Could you check a few things on this model? Use its own coordinates, in mm. A direction names the side the tool comes from. Coordinates: 2 decimals unless noted, no trailing zeros. Loops run counter-clockwise (first coordinate to the right, second up) from the corner with the lowest first, then second, coordinate; pieces in that order, holes last. Notation, with made-up numbers: (13.5, 2) - (22.5, 2) arc R20 cw to (22.5, 33) - close; hole circle Ø5 at (18.5, 87). An arc over 180 degrees is marked (long way). Use CSV: the item, a comma, the result in double quotes.
Autodesk Fusion 360 part; units mm, degrees
sketch "Sketch1" plane through (0, 0, 0) normal (0, 0, 1) x (1, 0, 0)
  line L0 (30, -30) -> (-30, -30)
  line L1 (-30, -30) -> (-30, 30)
  line L2 (-30, 30) -> (30, 30)
  line L3 (30, 30) -> (30, -30)
  line L4 (30, -30) -> (-30, 30) construction
  line L5 (-30, -30) -> (30, 30) construction
  dimension "d1" = 60
  dimension "d2" = 60
extrude "Extrude1" add sketch "Sketch1" along normal blind 6.35
sketch "Sketch2" plane through (0, 0, 6.35) normal (0, 0, 1) x (1, 0, 0)
  line L0 (30, 30) -> (-30, 30)
  line L1 (-30, 30) -> (-30, -30)
  line L2 (-30, -30) -> (30, -30)
  line L3 (30, -30) -> (30, 30)
  line L4 (20.5, -20.5) -> (-20.5, -20.5)
  line L5 (-20.5, -20.5) -> (-20.5, 20.5)
  line L6 (-20.5, 20.5) -> (20.5, 20.5)
  line L7 (20.5, 20.5) -> (20.5, -20.5)
  line L8 (20.5, -20.5) -> (-20.5, 20.5) construction
  line L9 (-20.5, -20.5) -> (20.5, 20.5) construction
  circle A0 centre (-20.5, 20.5) radius 3.575
  circle A1 centre (20.5, 20.5) radius 3.575
  circle A2 centre (20.5, -20.5) radius 2.5
  circle A3 centre (-20.5, -20.5) radius 2.5
  dimension "d5" = 41
  dimension "d6" = 41
  dimension "d7" = 7.15
  dimension "d8" = 7.15
  dimension "d9" = 5
  dimension "d10" = 5
extrude "Extrude2" cut sketch "Sketch2" against normal through all contours L4 L5 A3 | L4 L5 A3 | L4 L7 A2 | L4 L7 A2 | L5 L6 A0 | L5 L6 A0 | L6 L7 A1 | L6 L7 A1
sketch "Sketch3" plane through (0, 0, 6.35) normal (0, 0, 1) x (1, 0, 0)
  circle A0 centre (-20.5, -20.5) radius 2.5
  circle A1 centre (-20.5, 20.5) radius 3.575
  circle A2 centre (20.5, -20.5) radius 2.5
  circle A3 centre (20.5, 20.5) radius 3.575
  line L0 (30, 30) -> (-30, 30)
  line L1 (-30, 30) -> (-30, -30)
  line L2 (-30, -30) -> (30, -30)
  line L3 (30, -30) -> (30, 30)
  circle A4 centre (-20.5, -20.5) radius 5.05
  circle A5 centre (20.5, -20.5) radius 5.05
  circle A6 centre (20.5, 20.5) radius 5.05
  circle A7 centre (-20.5, 20.5) radius 5.05
  dimension "d12" = 10.1
  dimension "d13" = 10.1
  dimension "d14" = 10.1
  dimension "d15" = 10.1
extrude "Extrude3" cut sketch "Sketch3" against normal blind 2 contours A4 | A5 | A6 | A7
fillet "Fillet1" radius 5 2 edges at (30, -30, 3.175) (30, 30, 3.175)
fillet "Fillet2" radius 5 2 edges at (-30, 30, 3.175) (-30, -30, 3.175)
sketch "Sketch4" plane through (0, 0, 6.35) normal (0, 0, 1) x (1, 0, 0)
  arc A0 (-30, -25) -> (-25, -30) centre (-25, -25) ccw
  line L0 (-25, -30) -> (25, -30)
  arc A1 (25, -30) -> (30, -25) centre (25, -25) ccw
  line L1 (30, -25) -> (30, 25)
  arc A2 (30, 25) -> (25, 30) centre (25, 25) ccw
  line L2 (25, 30) -> (-25, 30)
  arc A3 (-25, 30) -> (-30, 25) centre (-25, 25) ccw
  line L3 (-30, 25) -> (-30, -25)
  circle A4 centre (20.5, 20.5) radius 5.05
  circle A5 centre (20.5, -20.5) radius 5.05
  circle A6 centre (-20.5, 20.5) radius 5.05
  circle A7 centre (-20.5, -20.5) radius 5.05
  circle A8 centre (0, 0) radius 2.5
  circle A9 centre (10, 0) radius 2.5
  circle A10 centre (-10, 0) radius 2.5
  line L4 (-25.75, -3.375) -> (-28.25, -3.375)
  line L5 (-28.25, -3.375) -> (-28.25, 3.375)
  line L6 (-28.25, 3.375) -> (-25.75, 3.375)
  line L7 (-25.75, 3.375) -> (-25.75, -3.375)
  line L8 (-25.75, -3.375) -> (-28.25, 3.375) construction
  line L9 (-28.25, -3.375) -> (-25.75, 3.375) construction
  line L10 (28.25, -3.375) -> (25.75, -3.375)
  line L11 (25.75, -3.375) -> (25.75, 3.375)
  line L12 (25.75, 3.375) -> (28.25, 3.375)
  line L13 (28.25, 3.375) -> (28.25, -3.375)
  line L14 (28.25, -3.375) -> (25.75, 3.375) construction
  line L15 (25.75, -3.375) -> (28.25, 3.375) construction
  point P0 (-27, 0)
  point P1 (27, 0)
  dimension "d20" = 5
  dimension "d21" = 5
  dimension "d22" = 5
  dimension "d23" = 6.75
  dimension "d24" = 2.5
  dimension "d25" = 6.75
  dimension "d26" = 2.5
extrude "Extrude4" cut sketch "Sketch4" against normal through all contours A8 | A9 | A10 | L4 L5 L6 L7 | L10 L11 L12 L13
sketch "Sketch5" plane through (0, 0, 6.35) normal (0, 0, 1) x (1, 0, 0)
  circle A0 centre (0, 0) radius 2.5
  circle A1 centre (-10, 0) radius 2.5
  circle A2 centre (10, 0) radius 2.5
  line L0 (-25.75, 3.375) -> (-25.75, -3.375)
  line L1 (-25.75, -3.375) -> (-28.25, -3.375)
  line L2 (-28.25, -3.375) -> (-28.25, 3.375)
  line L3 (-28.25, 3.375) -> (-25.75, 3.375)
  line L4 (28.25, 3.375) -> (28.25, -3.375)
  line L5 (28.25, -3.375) -> (25.75, -3.375)
  line L6 (25.75, -3.375) -> (25.75, 3.375)
  line L7 (25.75, 3.375) -> (28.25, 3.375)
  arc A3 (-30, -25) -> (-25, -30) centre (-25, -25) ccw
  line L8 (-25, -30) -> (25, -30)
  arc A4 (25, -30) -> (30, -25) centre (25, -25) ccw
  line L9 (30, -25) -> (30, 25)
  arc A5 (30, 25) -> (25, 30) centre (25, 25) ccw
  line L10 (25, 30) -> (-25, 30)
  arc A6 (-25, 30) -> (-30, 25) centre (-25, 25) ccw
  line L11 (-30, 25) -> (-30, -25)
  circle A7 centre (20.5, 20.5) radius 5.05
  circle A8 centre (20.5, -20.5) radius 5.05
  circle A9 centre (-20.5, 20.5) radius 5.05
  circle A10 centre (-20.5, -20.5) radius 5.05
  circle A11 centre (-20.5, 20.5) radius 6
  circle A12 centre (20.5, 20.5) radius 6
  dimension "d28" = 12
  dimension "d29" = 12
extrude "Extrude5" cut sketch "Sketch5" against normal blind 2 contours A11 | A12
sketch "Sketch6" plane through (0, 0, 6.35) normal (0, 0, 1) x (1, 0, 0)
  circle A0 centre (-20.5, 20.5) radius 6
  circle A1 centre (20.5, 20.5) radius 6
  circle A2 centre (0, 0) radius 2.5
  circle A3 centre (-10, 0) radius 2.5
  circle A4 centre (10, 0) radius 2.5
  line L0 (-25.75, 3.375) -> (-25.75, -3.375)
  line L1 (-25.75, -3.375) -> (-28.25, -3.375)
  line L2 (-28.25, -3.375) -> (-28.25, 3.375)
  line L3 (-28.25, 3.375) -> (-25.75, 3.375)
  line L4 (28.25, 3.375) -> (28.25, -3.375)
  line L5 (28.25, -3.375) -> (25.75, -3.375)
  line L6 (25.75, -3.375) -> (25.75, 3.375)
  line L7 (25.75, 3.375) -> (28.25, 3.375)
  arc A5 (-30, -25) -> (-25, -30) centre (-25, -25) ccw
  line L8 (-25, -30) -> (25, -30)
  arc A6 (25, -30) -> (30, -25) centre (25, -25) ccw
  line L9 (30, -25) -> (30, 25)
  arc A7 (30, 25) -> (25, 30) centre (25, 25) ccw
  line L10 (25, 30) -> (-25, 30)
  arc A8 (-25, 30) -> (-30, 25) centre (-25, 25) ccw
  line L11 (-30, 25) -> (-30, -25)
  circle A9 centre (20.5, -20.5) radius 5.05
  circle A10 centre (-20.5, -20.5) radius 5.05
  circle A11 centre (-20.5, 20.5) radius 3.65
  circle A12 centre (20.5, 20.5) radius 3.65
  dimension "d32" = 7.3
  dimension "d33" = 7.3
extrude "Extrude6" cut sketch "Sketch6" against normal through all contours A11
sketch "Sketch7" plane through (0, 0, 4.35) normal (0, 0, 1) x (1, 0, 0)
  circle A0 centre (20.5, 20.5) radius 6
  circle A1 centre (20.5, 20.5) radius 3.575
  circle A2 centre (20.5, 20.5) radius 3.65
  dimension "d35" = 7.3
extrude "Extrude7" cut sketch "Sketch7" against normal through all contours A2
move_face "OffsetFaces1" offset -1 1 faces at (-25.75, 1.125, 4.2333)
move_face "OffsetFaces2" offset 1 1 faces at (28.25, -1.125, 2.1167)
move_face "OffsetFaces3" offset 1 1 faces at (-28.25, 1.125, 2.1167)
move_face "OffsetFaces4" offset -1 1 faces at (25.75, 1.125, 2.1167)
sketch "Sketch9" plane through (0, 0, 6.35) normal (0, 0, 1) x (1, 0, 0)
  circle A0 centre (-20.5, 20.5) radius 6
  circle A1 centre (20.5, 20.5) radius 6
  circle A2 centre (0, 0) radius 2.5
  circle A3 centre (-10, 0) radius 2.5
  circle A4 centre (10, 0) radius 2.5
  line L0 (-24.75, 3.375) -> (-24.75, -3.375)
  line L1 (-24.75, -3.375) -> (-27.25, -3.375)
  line L2 (-27.25, -3.375) -> (-27.25, 3.375)
  line L3 (-27.25, 3.375) -> (-24.75, 3.375)
  line L4 (27.25, 3.375) -> (27.25, -3.375)
  line L5 (27.25, -3.375) -> (24.75, -3.375)
  line L6 (24.75, -3.375) -> (24.75, 3.375)
  line L7 (24.75, 3.375) -> (27.25, 3.375)
  arc A5 (-30, -25) -> (-25, -30) centre (-25, -25) ccw
  line L8 (-25, -30) -> (25, -30)
  arc A6 (25, -30) -> (30, -25) centre (25, -25) ccw
  line L9 (30, -25) -> (30, 25)
  arc A7 (30, 25) -> (25, 30) centre (25, 25) ccw
  line L10 (25, 30) -> (-25, 30)
  arc A8 (-25, 30) -> (-30, 25) centre (-25, 25) ccw
  line L11 (-30, 25) -> (-30, -25)
  circle A9 centre (20.5, -20.5) radius 5.05
  circle A10 centre (-20.5, -20.5) radius 5.05
  line L12 (-27.25, 3.375) -> (-30, 3.375)
  line L13 (-30, 3.375) -> (-30, -3.375)
  line L14 (-30, -3.375) -> (-27.25, -3.375)
  line L15 (-27.25, -3.375) -> (-27.25, 3.375)
  circle A11 centre (-0.0171, 20.5) radius 3.625
  dimension "d48" = 6.75
  dimension "d51" = 7.25
extrude "Extrude9" cut sketch "Sketch9" against normal blind 1.75 contours L2 L11 L12 L13 L14 L15
sketch "Sketch10" plane through (0, 0, 6.35) normal (0, 0, 1) x (1, 0, 0)
  line L0 (-30, -3.375) -> (-30, -25)
  arc A0 (-30, -25) -> (-25, -30) centre (-25, -25) ccw
  line L1 (-25, -30) -> (25, -30)
  arc A1 (25, -30) -> (30, -25) centre (25, -25) ccw
  line L2 (30, -25) -> (30, 25)
  arc A2 (30, 25) -> (25, 30) centre (25, 25) ccw
  line L3 (25, 30) -> (-25, 30)
  arc A3 (-25, 30) -> (-30, 25) centre (-25, 25) ccw
  line L4 (-30, 25) -> (-30, 3.375)
  line L5 (-30, 3.375) -> (-24.75, 3.375)
  line L6 (-24.75, 3.375) -> (-24.75, -3.375)
  line L7 (-24.75, -3.375) -> (-30, -3.375)
  circle A4 centre (-20.5, 20.5) radius 6
  circle A5 centre (20.5, 20.5) radius 6
  circle A6 centre (0, 0) radius 2.5
  circle A7 centre (-10, 0) radius 2.5
  circle A8 centre (10, 0) radius 2.5
  line L8 (27.25, 3.375) -> (27.25, -3.375)
  line L9 (27.25, -3.375) -> (24.75, -3.375)
  line L10 (24.75, -3.375) -> (24.75, 3.375)
  line L11 (24.75, 3.375) -> (27.25, 3.375)
  circle A9 centre (20.5, -20.5) radius 5.05
  circle A10 centre (-20.5, -20.5) radius 5.05
  line L12 (27.25, 3.375) -> (30, 3.375)
  line L13 (30, 3.375) -> (30, -3.375)
  line L14 (30, -3.375) -> (27.25, -3.375)
  line L15 (27.25, -3.375) -> (27.25, 3.375)
  dimension "d45" = 6.75
extrude "Extrude10" cut sketch "Sketch10" against normal blind 1.75 contours L2 L8 L12 L13 L14 L15
extrude "Extrude11" cut sketch "Sketch9" against normal blind 1.75 contours L2 L11 L12 L13 L14 L15
extrude "Extrude12" cut sketch "Sketch9" against normal through all contours A11
sketch "Sketch11" plane through (0, 0, 6.35) normal (0, 0, 1) x (1, 0, 0)
  circle A0 centre (-0.0171, 20.5) radius 3.625
  line L0 (30, -3.375) -> (24.75, -3.375)
  line L1 (24.75, -3.375) -> (24.75, 3.375)
  line L2 (24.75, 3.375) -> (30, 3.375)
  line L3 (30, 3.375) -> (30, 25)
  arc A1 (30, 25) -> (25, 30) centre (25, 25) ccw
  line L4 (25, 30) -> (-25, 30)
  arc A2 (-25, 30) -> (-30, 25) centre (-25, 25) ccw
  line L5 (-30, 25) -> (-30, 3.375)
  line L6 (-30, 3.375) -> (-24.75, 3.375)
  line L7 (-24.75, 3.375) -> (-24.75, -3.375)
  line L8 (-24.75, -3.375) -> (-30, -3.375)
  line L9 (-30, -3.375) -> (-30, -25)
  arc A3 (-30, -25) -> (-25, -30) centre (-25, -25) ccw
  line L10 (-25, -30) -> (25, -30)
  arc A4 (25, -30) -> (30, -25) centre (25, -25) ccw
  line L11 (30, -25) -> (30, -3.375)
  circle A5 centre (-20.5, -20.5) radius 5.05
  circle A6 centre (20.5, -20.5) radius 5.05
  circle A7 centre (10, 0) radius 2.5
  circle A8 centre (-10, 0) radius 2.5
  circle A9 centre (0, 0) radius 2.5
  circle A10 centre (20.5, 20.5) radius 6
  circle A11 centre (-20.5, 20.5) radius 6
  circle A12 centre (-0.0171, 20.5) radius 6
  dimension "d53" = 12
extrude "Extrude13" cut sketch "Sketch11" against normal blind 2 contours A12
sketch "Sketch12" plane through (0, 0, 6.35) normal (0, 0, 1) x (1, 0, 0)
  circle A0 centre (-0.0171, 20.5) radius 6
  line L0 (30, -3.375) -> (24.75, -3.375)
  line L1 (24.75, -3.375) -> (24.75, 3.375)
  line L2 (24.75, 3.375) -> (30, 3.375)
  line L3 (30, 3.375) -> (30, 25)
  arc A1 (30, 25) -> (25, 30) centre (25, 25) ccw
  line L4 (25, 30) -> (-25, 30)
  arc A2 (-25, 30) -> (-30, 25) centre (-25, 25) ccw
  line L5 (-30, 25) -> (-30, 3.375)
  line L6 (-30, 3.375) -> (-24.75, 3.375)
  line L7 (-24.75, 3.375) -> (-24.75, -3.375)
  line L8 (-24.75, -3.375) -> (-30, -3.375)
  line L9 (-30, -3.375) -> (-30, -25)
  arc A3 (-30, -25) -> (-25, -30) centre (-25, -25) ccw
  line L10 (-25, -30) -> (25, -30)
  arc A4 (25, -30) -> (30, -25) centre (25, -25) ccw
  line L11 (30, -25) -> (30, -3.375)
  circle A5 centre (-20.5, -20.5) radius 5.05
  circle A6 centre (20.5, -20.5) radius 5.05
  circle A7 centre (10, 0) radius 2.5
  circle A8 centre (-10, 0) radius 2.5
  circle A9 centre (0, 0) radius 2.5
  circle A10 centre (20.5, 20.5) radius 6
  circle A11 centre (-20.5, 20.5) radius 6
(1) Suppose I cut it at D-D (z = 3). State how many separate pieces and enclosed holes the cut face has, plus the area to 3 significant figures.
Computed:
separate pieces,"1"
enclosed holes,"10"
area,"3,320 mm²"
(2) Suppose I cut it at A-A (x = -20.5). Write out the boundary of the cut face in (y, z), plus the area to 3 significant figures.
Computed:
outline,"(-30, 0) - (-23, 0) - (-23, 4.35) - (-25.55, 4.35) - (-25.55, 6.35) - (-30, 6.35) - close; (-18, 0) - (16.85, 0) - (16.85, 4.35) - (14.5, 4.35) - (14.5, 6.35) - (-15.45, 6.35) - (-15.45, 4.35) - (-18, 4.35) - close; (24.15, 0) - (30, 0) - (30, 6.35) - (26.5, 6.35) - (26.5, 4.35) - (24.15, 4.35) - close"
area,"283 mm²"
(3) Which directions (+Z, -Z, +X, -X, +Y, -Y) give clear straight access to the entire face, cutting with the end or side of a thin tool? Please do faces 5 (the face through (0, -6, 6.35)), 6 (the face through (18, -22, 4.35)), 7 (the face through (-29, 0, 4.6)), 8 (the face through (27.25, 0, 2)), 9 (the face through (29, 0, 4.6)).
Computed:
face 5,"+Z, +X, -X, +Y, -Y"
face 6,"+Z"
face 7,"+Z, -X"
face 8,"+Z, -Z"
face 9,"+Z, +X"
(4) Suppose I cut it at B-B (x = -10). Write out the boundary of the cut face in (y, z).
Computed:
outline,"(-30, 0) - (-2.5, 0) - (-2.5, 6.35) - (-30, 6.35) - close; (2.5, 0) - (30, 0) - (30, 6.35) - (2.5, 6.35) - close"
(5) Thinking about a two-plate mould opening in Y: for faces 1 (the face through (0, 30, 3)), 2 (the face through (28, -29, 3)), 3 (the face through (1.656, 17.284, 2.205)), 4 (the face through (-30, 0, 3)), which applies, +Y half, -Y half, draft (parallel to the pull), parting line (faces both ways), or undercut?
Computed:
face 1,"+Y half"
face 2,"-Y half"
face 3,"undercut"
face 4,"draft"
(6) Suppose I cut it at C-C (y = 20.5). Write out the boundary of the cut face in (x, z), plus the area to 3 significant figures.
Computed:
outline,"(-30, 0) - (-24.15, 0) - (-24.15, 4.35) - (-26.5, 4.35) - (-26.5, 6.35) - (-30, 6.35) - close; (-16.85, 0) - (-3.64, 0) - (-3.64, 4.35) - (-6.02, 4.35) - (-6.02, 6.35) - (-14.5, 6.35) - (-14.5, 4.35) - (-16.85, 4.35) - close; (3.61, 0) - (16.85, 0) - (16.85, 4.35) - (14.5, 4.35) - (14.5, 6.35) - (5.98, 6.35) - (5.98, 4.35) - (3.61, 4.35) - close; (24.15, 0) - (30, 0) - (30, 6.35) - (26.5, 6.35) - (26.5, 4.35) - (24.15, 4.35) - close"
area,"214 mm²"
(7) Will these pins go through, and if not, where does the flat tip stop? pin 1 (14 mm diameter, centred on x = -0.02, y = 20.5, fed in from +Z); pin 2 (1.6 mm diameter, centred on x = 26, z = 3.5, fed in from +Y); pin 3 (3 mm diameter, centred on x = -21, y = -18.5, fed in from +Z); pin 4 (2 mm diameter, centred on x = 28, y = 1.5, fed in from +Z).
Computed:
pin 1,"stops at z = 6.35"
pin 2,"stops at y = 30"
pin 3,"stops at z = 4.35"
pin 4,"stops at z = 4.6"
(8) Please list where these lines run through material, in increasing order: line 1 (X direction, y = -19, z = 1.25); line 2 (X direction, y = -1, z = 2); line 3 (X direction, y = -20, z = 1.75).
Computed:
line 1,"x = -30 to -22.5, -18.5 to 18.5, 22.5 to 30"
line 2,"x = -30 to -27.25, -24.75 to -12.29, -7.71 to -2.29, 2.29 to 7.71, 12.29 to 24.75, 27.25 to 30"
line 3,"x = -30 to -22.95, -18.05 to 18.05, 22.95 to 30"
